Part model, mm, in its own coordinate system. Give positions to 0.01 mm unless a question says otherwise; leave off trailing zeros. Loops run counter-clockwise (first coordinate to the right, second up) from the corner with the lowest first, then second, coordinate; pieces in that order, holes last. Notation, with made-up numbers: M 83.25,85.5 L 122.25,85.5 A16 ccw 122.25,92.5 Z; hole C 43,72.25 d1. An arc over 180 degrees is marked long. Put each result on its own line as item: value. Start each with the question number.
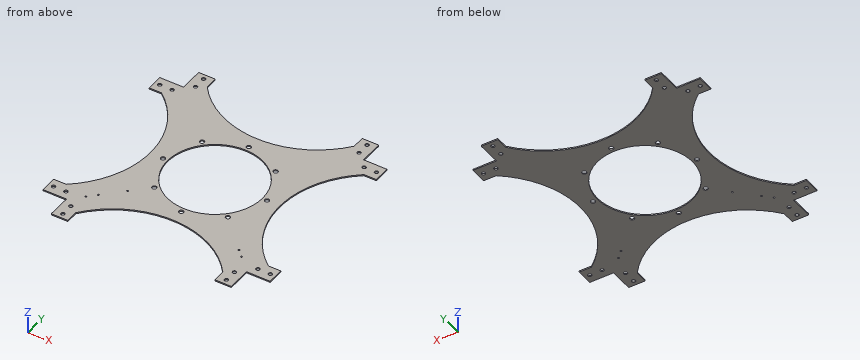
```python
from build123d import *

# Parameters (mm, degrees)
SKETCH1_R          = 114.5
BASE_FLANGE1_DEPTH = 3
SKETCH2_R          = 4.6
EXTRUDE1_DEPTH     = 3
SKETCH3_R          = 5.5
EXTRUDE2_DEPTH     = 3
CIRPATTERN1_COUNT  = 8
SKETCH4_R          = 2.1
CUT_EXTRUDE1_DEPTH = 10


# Sheet-metal steps are written as plain solids
with BuildPart() as part:
    # Sketch1 → Base-Flange1 (new body)
    with BuildSketch(Plane.XY):
        with BuildLine():
            Line((218, 218), (218, 275))
            Line((218, 275), (178, 275))
            Line((178, 275), (178, 245))
            ThreePointArc((178, 245), (0, 157.626305625), (-178, 245))
            Line((-178, 245), (-178, 275))
            Line((-178, 275), (-218, 275))
            Line((-218, 275), (-218, 218))
            Line((-218, 218), (-275, 218))
            Line((-275, 218), (-275, 178))
            Line((-275, 178), (-245, 178))
            ThreePointArc((-245, 178), (-157.626305625, 0), (-245, -178))
            Line((-245, -178), (-275, -178))
            Line((-275, -178), (-275, -218))
            Line((-275, -218), (-218, -218))
            Line((-218, -218), (-218, -275))
            Line((-218, -275), (-178, -275))
            Line((-178, -275), (-178, -245))
            ThreePointArc((-178, -245), (0, -157.626305625), (178, -245))
            Line((178, -245), (178, -275))
            Line((178, -275), (218, -275))
            Line((218, -275), (218, -218))
            Line((218, -218), (275, -218))
            Line((275, -218), (275, -178))
            Line((275, -178), (245, -178))
            ThreePointArc((245, -178), (157.626305625, 0), (245, 178))
            Line((245, 178), (275, 178))
            Line((275, 178), (275, 218))
            Line((275, 218), (218, 218))
        make_face()
        Circle(SKETCH1_R, mode=Mode.SUBTRACT)
    extrude(amount=BASE_FLANGE1_DEPTH)

    # Sketch2 → Extrude1 (cut)
    with BuildSketch(Plane.XY.offset(3)):
        with Locations((198, 262.5)):
            Circle(SKETCH2_R)
        with Locations((198, 232.5)):
            Circle(SKETCH2_R)
        with Locations((232.5, 198)):
            Circle(SKETCH2_R)
        with Locations((262.5, 198)):
            Circle(SKETCH2_R)
        with Locations(Location((262.5, -198, 0), (0, 0, 180))):
            Circle(SKETCH2_R)
        with Locations(Location((232.5, -198, 0), (0, 0, 180))):
            Circle(SKETCH2_R)
        with Locations(Location((198, -232.5, 0), (0, 0, 180))):
            Circle(SKETCH2_R)
        with Locations(Location((198, -262.5, 0), (0, 0, 180))):
            Circle(SKETCH2_R)
        with Locations((-198, -262.5)):
            Circle(SKETCH2_R)
        with Locations((-198, -232.5)):
            Circle(SKETCH2_R)
        with Locations((-232.5, -198)):
            Circle(SKETCH2_R)
        with Locations((-262.5, -198)):
            Circle(SKETCH2_R)
        with Locations(Location((-262.5, 198, 0), (0, 0, 180))):
            Circle(SKETCH2_R)
        with Locations(Location((-232.5, 198, 0), (0, 0, 180))):
            Circle(SKETCH2_R)
        with Locations(Location((-198, 232.5, 0), (0, 0, 180))):
            Circle(SKETCH2_R)
        with Locations(Location((-198, 262.5, 0), (0, 0, 180))):
            Circle(SKETCH2_R)
    extrude(amount=-EXTRUDE1_DEPTH, mode=Mode.SUBTRACT)

    # Sketch3 → Extrude2 (cut)
    with BuildSketch(Plane.XY.offset(3)):
        with Locations((0, 126)):
            Circle(SKETCH3_R)
    extrude2 = extrude(amount=-EXTRUDE2_DEPTH, mode=Mode.SUBTRACT)

    # CirPattern1: Extrude2 ×8 about axis
    cirpattern1_axis = Axis((0, 0, 0), (0, 0, 1))
    for i in range(1, CIRPATTERN1_COUNT):
        add(extrude2.rotate(cirpattern1_axis, i * 360 / CIRPATTERN1_COUNT), mode=Mode.SUBTRACT)

    # Sketch4 → Cut-Extrude1 (cut)
    with BuildSketch(Plane.XY.offset(3)):
        with Locations((-189.715728753, -189.715728753)):
            Circle(SKETCH4_R)
        with Locations((-171.330952442, -171.330952442)):
            Circle(SKETCH4_R)
        with Locations((-128.197438789, -128.197438789)):
            Circle(SKETCH4_R)
        with Locations((166.381204973, -166.381204973)):
            Circle(SKETCH4_R)
        with Locations((182.644660941, -182.644660941)):
            Circle(SKETCH4_R)
    extrude(amount=-CUT_EXTRUDE1_DEPTH, mode=Mode.SUBTRACT)


solid = part.part
```
1) Wall check: L1, parallel to Y at x = -0.5, z = 1.55; L2, parallel to Y at x = -262.5, z = 1.5; L3, parallel to X at y = 235.5, z = 1.25. Give the ranges that are in metal, low to high.
2) Pin check, flat tips, straight feed: pin 1 Ø0.9 at (y, z) = (263.5, 2) entering from +X; pin 2 Ø4 at (x, y) = (-189.72, -189.72) entering from -Z; pin 3 Ø1.5 at (x, z) = (-52, 2.5) entering from -Y; pin 4 Ø1.5 at (x, z) = (150.5, 2) entering from -Y. Stop position of each tip, or through.
3) Band-saw the part on A-A on y = -16. Give the cut face in (x, z), then the cut area to 3 significant figures.
4) Band-saw the part on B-B on x = 53.5. Give the cut face in (y, z), then the cut area to 3 significant figures.
5) Band-saw the part on C-C on z = 2.35. State how many separate pieces and enclosed holes the cut face has, then the cut area to 3 significant figures.
Evaluation:
1. L1: -157.63 to -131.48, -120.52 to -114.5, 114.5 to 120.52, 131.48 to 157.63
1. L2: -218 to -202.6, -193.4 to -178, 178 to 193.4, 202.6 to 218
1. L3: -218 to -201.49, -194.51 to -170.23, 170.23 to 194.51, 201.49 to 218
2. pin 1: x = 218
2. pin 2: through
2. pin 3: y = -163.9
2. pin 4: y = -216.05
3. outline: M -158.2,0 L -113.38,0 L -113.38,3 L -158.2,3 Z; M 113.38,0 L 158.2,0 L 158.2,3 L 113.38,3 Z
3. area: 269 mm2
4. outline: M -164.08,0 L -101.23,0 L -101.23,3 L -164.08,3 Z; M 101.23,0 L 164.08,0 L 164.08,3 L 101.23,3 Z
4. area: 377 mm2
5. separate pieces: 1
5. enclosed holes: 30
5. area: 117,000 mm2
